from build123d import *

# Parameters (mm, degrees)
SKETCH1_W                               = 12
SKETCH1_H                               = 75
BASE_DEPTH                              = 500
SKETCH2_W                               = 99
SKETCH2_H                               = 25
LAP_JOINT_CUTOUT_DEPTH                  = 506.736097189
LAP_JOINT_BOLT_HOLE_PATTERN_D           = 5.5
LAP_JOINT_BOLT_HOLE_PATTERN_CBORE_D     = 10
LAP_JOINT_BOLT_HOLE_PATTERN_CBORE_DEPTH = 5
CHAMFER_FRONT_SIZE                      = 150
CHAMFER_FRONT_SIZE2                     = 54.59553514
CHAMFER_REAR_SIZE                       = 150
CHAMFER_REAR_SIZE2                      = 54.59553514
BREAK_CHAMFER_CORNERS_R                 = 20
CROSS_TIE_BOLT_HOLE_PATTERN_D           = 5.5
CROSS_TIE_BOLT_HOLE_PATTERN_CBORE_D     = 10
CROSS_TIE_BOLT_HOLE_PATTERN_CBORE_DEPTH = 5


with BuildPart() as part:
    # Sketch1 → base (new body)
    with BuildSketch(Plane.XY):
        with Locations((6, 37.5)):
            Rectangle(SKETCH1_W, SKETCH1_H)
    extrude(amount=BASE_DEPTH)

    # Sketch2 → lap joint cutout (cut, through all)
    with BuildSketch(Plane.ZY):
        with Locations((250, 62.5)):
            Rectangle(SKETCH2_W, SKETCH2_H)
    extrude(amount=-LAP_JOINT_CUTOUT_DEPTH, mode=Mode.SUBTRACT)

    # lap joint bolt hole pattern (through all)
    with Locations(Plane(origin=(12, 0, 0), x_dir=(0, 0, -1), z_dir=(1, 0, 0))):
        with Locations((-293.5, 40), (-206.5, 10), (-293.5, 10), (-206.5, 40)):
            CounterBoreHole(LAP_JOINT_BOLT_HOLE_PATTERN_D / 2, LAP_JOINT_BOLT_HOLE_PATTERN_CBORE_D / 2, LAP_JOINT_BOLT_HOLE_PATTERN_CBORE_DEPTH)

    # chamfer front
    chamfer_front_edges = [part.edges().sort_by_distance(p)[0] for p in [
        (6, 75, 0),
    ]]
    chamfer_front_side = [part.faces().sort_by_distance(p)[0] for p in [
        (6, 75, 100.25),
    ]]
    chamfer(chamfer_front_edges, length=CHAMFER_FRONT_SIZE, length2=CHAMFER_FRONT_SIZE2, reference=chamfer_front_side[0])

    # chamfer rear
    chamfer_rear_edges = [part.edges().sort_by_distance(p)[0] for p in [
        (6, 75, 500),
    ]]
    chamfer_rear_side = [part.faces().sort_by_distance(p)[0] for p in [
        (6, 75, 399.75),
    ]]
    chamfer(chamfer_rear_edges, length=CHAMFER_REAR_SIZE, length2=CHAMFER_REAR_SIZE2, reference=chamfer_rear_side[0])

    # break chamfer corners
    break_chamfer_corners_edges = [part.edges().sort_by_distance(p)[0] for p in [
        (6, 20.40446486, 0),
        (6, 20.40446486, 500),
    ]]
    fillet(break_chamfer_corners_edges, radius=BREAK_CHAMFER_CORNERS_R)

    # cross tie bolt hole pattern (through all)
    with Locations(Plane(origin=(12, 0, 0), x_dir=(0, 0, -1), z_dir=(1, 0, 0))):
        with Locations((-305.5, 40), (-305.5, 10)):
            cross_tie_bolt_hole_pattern = CounterBoreHole(CROSS_TIE_BOLT_HOLE_PATTERN_D / 2, CROSS_TIE_BOLT_HOLE_PATTERN_CBORE_D / 2, CROSS_TIE_BOLT_HOLE_PATTERN_CBORE_DEPTH)

    # mirror cross tie bolt hole pattern: cross tie bolt hole pattern across plane
    add(cross_tie_bolt_hole_pattern.mirror(Plane(origin=(0, 0, 250), x_dir=(1, 0, 0), z_dir=(0, 0, -1))), mode=Mode.SUBTRACT)


solid = part.part
Source: CAD feature listing. Evaluate the final solid. Frame: model axes, mm. A direction names the side the tool comes from. Coordinates: 2 decimals unless noted, no trailing zeros. Order: outer loops, then holes, each group sorted by start corner. A loop starts at its lowest first (then second) coordinate and runs counter-clockwise, first axis right, second up.
Item 1: Set-up query: faces 5 (the face through (6, 62, 299.5)), 6 (the face through (5.916, 49.748, 80.622)), 7 (the face through (9.54, 11.5, 288.73)). Return all of +Z, -Z, +X, -X, +Y, -Y with unobstructed straight access to the full face (end or side cutting, diameter ignored); none if empty.
Output values:
face 5: +X, -X, +Y
face 6: -Z, +X, -X, +Y
face 7: +X
Item 2: Cut plane B-B (y = 58.5). Return loops of the section in (x, z).
Output values:
outline: (0, 104.67) - (12, 104.67) - (12, 200.5) - (0, 200.5) - close; (0, 299.5) - (12, 299.5) - (12, 395.33) - (0, 395.33) - close
Item 3: First-contact query: P1, Ø11, axis at y = 41, z = 207, coming from the +X side; P2, Ø7, axis at y = 10, z = 206.5, coming from the +X side. Flat tips, straight axial feed; report the tip coordinate or a pass-through.
Output values:
P1: stops at x = 12
P2: stops at x = 7
Item 4: Material intervals for line 1 (Y direction, x = 10.45, z = 305.5); line 2 (Y direction, x = 2.75, z = 206.5); line 3 (Z direction, x = 9.25, y = 6.5), sorted ascending.
Output values:
line 1: y = 0 to 5, 15 to 35, 45 to 75
line 2: y = 0 to 7.25, 12.75 to 37.25, 42.75 to 50
line 3: z = 0 to 190.93, 198.07 to 202.93, 210.07 to 289.93, 297.07 to 301.93, 309.07 to 500
Item 5: Cut plane C-C (z = 417.5). Return loops of the section in (x, y).
Output values:
outline: (0, 0) - (12, 0) - (12, 50.43) - (0, 50.43) - close
Item 6: Pull-direction query (Z, two-part tool) for faces 1 (the face through (6, 75, 324)), 2 (the face through (6.1, 17.7, 3.5)), 3 (the face through (6.1, 17.7, 496.5)), 4 (the face through (9.535, 10.22, 189.505)); classes: pulls with the +Z half, pulls with the -Z half, needs draft (parallel to the pull), parting line crosses it, or undercut.
Output values:
face 1: needs draft
face 2: pulls with the -Z half
face 3: pulls with the +Z half
face 4: undercut
Item 7: Cut plane A-A (x = 2.25). Count the separate pieces of the cut face and the enclosed holes in it, plus the area to 3 significant figures.
Output values:
separate pieces: 1
enclosed holes: 8
area: 26,600 mm2
